Geometry check sheet. Reference: drawing and pictorial views, mm from the part's lowest x, y, z. Round coordinates to 2 decimals unless told otherwise and drop trailing zeros. Write each loop counter-clockwise with the first axis right and the second up, starting at its lowest first coordinate (ties: lowest second). Pieces come first, ordered by that corner, then holes. Notation, with made-up numbers: (-40, 12.5) -> (1, 12.5) arc R19 cw to (1, 18.5) -> close; hole circle Ø8 at (50.5, 89). An arc over 180 degrees is marked (long way). Answer as a JSON object with one key per item and string values. Group by question number.
(1) Gauge pin test, flat ends, axial feed: pin 1 Ø1 at (x, y) = (1, 1) entering from +Z; pin 2 Ø0.6 at (x, y) = (1, 14.5) entering from -Z; pin 3 Ø0.8 at (x, z) = (1, 1.5) entering from +Y. Record the tip position at first contact, or that the pin passes through.
(2) Sectioned sample at A-A on x = 1.9. Record the cut outline in (y, z), and give its area (3 significant figures).
(3) Scan lines: L1, parallel to Y at x = 0.45, z = 55; L2, parallel to Z at x = 0.25, y = 15.5; L3, parallel to Z at x = 0.45, y = 1. Record each from-to range of solid material in increasing order. Write a range as from..to.
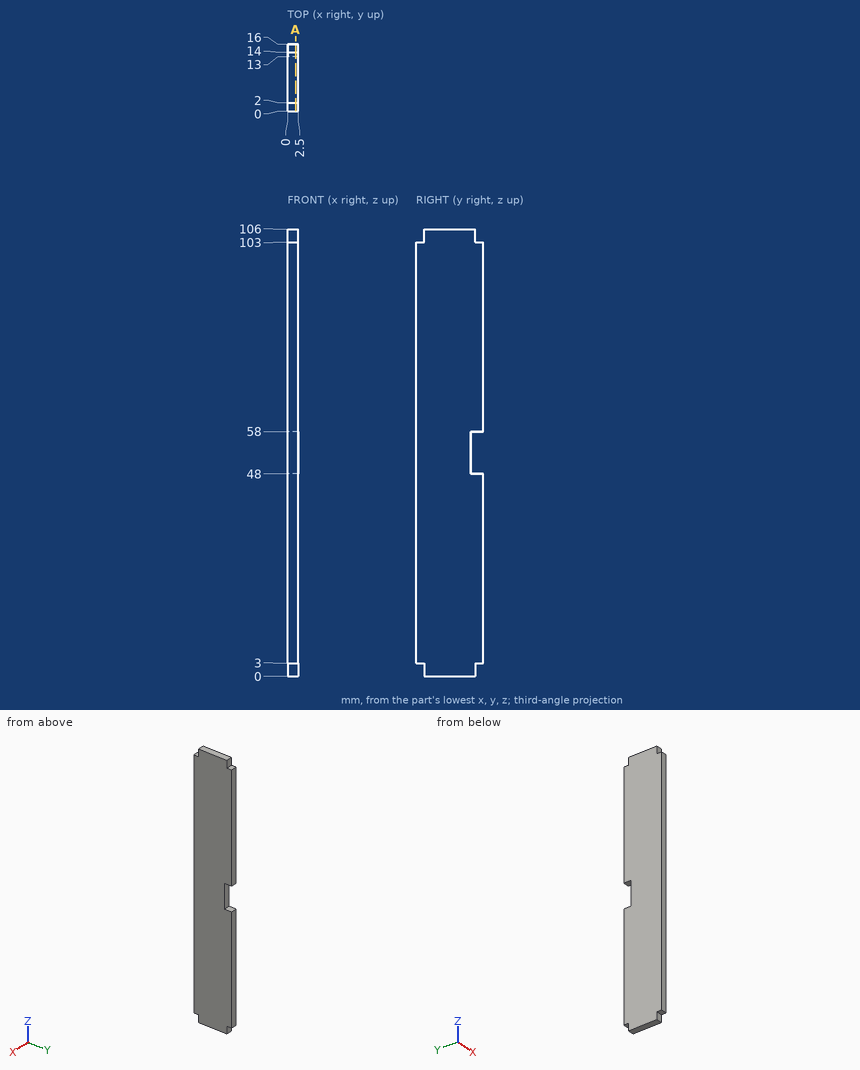
Computed values:
{
 "1": {"pin 1": "z = 103", "pin 2": "z = 3", "pin 3": "y = 14"},
 "2": {"outline": "(0, 3) -> (2, 3) -> (2, 0) -> (14, 0) -> (14, 3) -> (16, 3) -> (16, 48) -> (13, 48) -> (13, 58) -> (16, 58) -> (16, 103) -> (14, 103) -> (14, 106) -> (2, 106) -> (2, 103) -> (0, 103) -> close", "area": "1,640 mm2"},
 "3": {"L1": "0..13", "L2": "3..48, 58..103", "L3": "3..103"}
}
